```python
from build123d import *

# Parameters (mm, degrees)
SKETCH_1_R      = 2.1
EXTRUDE_1_DEPTH = 10


with BuildPart() as part:
    # 스케치1 → 보스-돌출1 (new body)
    with BuildSketch(Plane(origin=(0, 0, 0), x_dir=(1, 0, 0), z_dir=(0, 1, 0))):
        with BuildLine():
            Line((2, -4), (-2, -4))
            Line((-2, -4), (-5, -7))
            Line((-5, -7), (-5, -7.5))
            ThreePointArc((-5, -7.5), (-4.853553391, -7.853553391), (-4.5, -8))
            Line((-4.5, -8), (-3.1, -8))
            ThreePointArc((-3.1, -8), (-2.746446609, -8.146446609), (-2.6, -8.5))
            Line((-2.6, -8.5), (-2.6, -9.5))
            Line((-2.6, -9.5), (-3.1, -9.5))
            Line((-3.1, -9.5), (-3.1, -10))
            Line((-3.1, -10), (-9, -10))
            ThreePointArc((-9, -10), (-9.382683432, -9.923879533), (-9.707106781, -9.707106781))
            ThreePointArc((-9.707106781, -9.707106781), (-9.923879533, -9.382683432), (-10, -9))
            Line((-10, -9), (-10, -3.1))
            Line((-10, -3.1), (-9.5, -3.1))
            Line((-9.5, -3.1), (-9.5, -2.6))
            Line((-9.5, -2.6), (-8.5, -2.6))
            ThreePointArc((-8.5, -2.6), (-8.146446609, -2.746446609), (-8, -3.1))
            Line((-8, -3.1), (-8, -4.5))
            ThreePointArc((-8, -4.5), (-7.853553391, -4.853553391), (-7.5, -5))
            Line((-7.5, -5), (-7, -5))
            Line((-7, -5), (-4, -2))
            Line((-4, -2), (-4, 2))
            Line((-4, 2), (-7, 5))
            Line((-7, 5), (-7.5, 5))
            ThreePointArc((-7.5, 5), (-7.853553391, 4.853553391), (-8, 4.5))
            Line((-8, 4.5), (-8, 3.1))
            ThreePointArc((-8, 3.1), (-8.146446609, 2.746446609), (-8.5, 2.6))
            Line((-8.5, 2.6), (-9.5, 2.6))
            Line((-9.5, 2.6), (-9.5, 3.1))
            Line((-9.5, 3.1), (-10, 3.1))
            Line((-10, 3.1), (-10, 9))
            ThreePointArc((-10, 9), (-9.923879533, 9.382683432), (-9.707106781, 9.707106781))
            ThreePointArc((-9.707106781, 9.707106781), (-9.382683432, 9.923879533), (-9, 10))
            Line((-9, 10), (-3.1, 10))
            Line((-3.1, 10), (-3.1, 9.5))
            Line((-3.1, 9.5), (-2.6, 9.5))
            Line((-2.6, 9.5), (-2.6, 8.5))
            ThreePointArc((-2.6, 8.5), (-2.746446609, 8.146446609), (-3.1, 8))
            Line((-3.1, 8), (-4.5, 8))
            ThreePointArc((-4.5, 8), (-4.853553391, 7.853553391), (-5, 7.5))
            Line((-5, 7.5), (-5, 7))
            Line((-5, 7), (-2, 4))
            Line((-2, 4), (2, 4))
            Line((2, 4), (5, 7))
            Line((5, 7), (5, 7.5))
            ThreePointArc((5, 7.5), (4.853553391, 7.853553391), (4.5, 8))
            Line((4.5, 8), (3.1, 8))
            ThreePointArc((3.1, 8), (2.746446609, 8.146446609), (2.6, 8.5))
            Line((2.6, 8.5), (2.6, 9.5))
            Line((2.6, 9.5), (3.1, 9.5))
            Line((3.1, 9.5), (3.1, 10))
            Line((3.1, 10), (9, 10))
            ThreePointArc((9, 10), (9.382683432, 9.923879533), (9.707106781, 9.707106781))
            ThreePointArc((9.707106781, 9.707106781), (9.923879533, 9.382683432), (10, 9))
            Line((10, 9), (10, 3.1))
            Line((10, 3.1), (9.5, 3.1))
            Line((9.5, 3.1), (9.5, 2.6))
            Line((9.5, 2.6), (8.5, 2.6))
            ThreePointArc((8.5, 2.6), (8.146446609, 2.746446609), (8, 3.1))
            Line((8, 3.1), (8, 4.5))
            ThreePointArc((8, 4.5), (7.853553391, 4.853553391), (7.5, 5))
            Line((7.5, 5), (7, 5))
            Line((7, 5), (4, 2))
            Line((4, 2), (4, -2))
            Line((4, -2), (7, -5))
            Line((7, -5), (7.5, -5))
            ThreePointArc((7.5, -5), (7.853553391, -4.853553391), (8, -4.5))
            Line((8, -4.5), (8, -3.1))
            ThreePointArc((8, -3.1), (8.146446609, -2.746446609), (8.5, -2.6))
            Line((8.5, -2.6), (9.5, -2.6))
            Line((9.5, -2.6), (9.5, -3.1))
            Line((9.5, -3.1), (10, -3.1))
            Line((10, -3.1), (10, -9))
            ThreePointArc((10, -9), (9.923879533, -9.382683432), (9.707106781, -9.707106781))
            ThreePointArc((9.707106781, -9.707106781), (9.382683432, -9.923879533), (9, -10))
            Line((9, -10), (3.1, -10))
            Line((3.1, -10), (3.1, -9.5))
            Line((3.1, -9.5), (2.6, -9.5))
            Line((2.6, -9.5), (2.6, -8.5))
            ThreePointArc((2.6, -8.5), (2.746446609, -8.146446609), (3.1, -8))
            Line((3.1, -8), (4.5, -8))
            ThreePointArc((4.5, -8), (4.853553391, -7.853553391), (5, -7.5))
            Line((5, -7.5), (5, -7))
            Line((5, -7), (2, -4))
        make_face()
        Circle(SKETCH_1_R, mode=Mode.SUBTRACT)
    extrude(amount=EXTRUDE_1_DEPTH)


solid = part.part
```
Model file for the job. Use its own axes, mm. A direction names the side the tool comes from. Coordinates: 2 decimals unless noted, no trailing zeros. Loops run counter-clockwise (first coordinate to the right, second up) from the corner with the lowest first, then second, coordinate; pieces in that order, holes last. Notation, with made-up numbers: (44.25, 70) -> (85.25, 70) arc R22 ccw to (85.25, 93) -> close; hole circle Ø8 at (42.25, -28). An arc over 180 degrees is marked (long way). Answer as a JSON object with one key per item and string values.
Q1. Cut at B-B (x = 1.25). List the corners of the cut face in (y, z).
Report:
{"outline": "(0, -4) -> (10, -4) -> (10, -1.69) -> (0, -1.69) -> close; (0, 1.69) -> (10, 1.69) -> (10, 4) -> (0, 4) -> close"}
Q2. Probe probe 1 along X at (y, z) = (5.25, 0); probe 2 along X at (y, z) = (2, -3.25). List the from-to ranges inside material, lowest first.
Report:
{"probe 1": "x = -4 to -2.1, 2.1 to 4", "probe 2": "x = -10 to -8, -5.25 to 5.25, 8 to 10"}
Q3. Cut at A-A (z = 5.5). List the corners of the cut face in (x, y), and give its area (3 significant figures).
Report:
{"outline": "(-10, 0) -> (-3.5, 0) -> (-3.5, 10) -> (-10, 10) -> close; (3.5, 0) -> (10, 0) -> (10, 10) -> (3.5, 10) -> close", "area": "130 mm2"}
Q4. 3-axis set-ups, long thin cutter, end or side, ignore diameter. For faces 4 (the flat face through (9, 5, 2.6)), 5 (the flat face through (-4, 5, 8)), 6 (the flat face through (0, 5, -4)): which of +Z, -Z, +X, -X, +Y, -Y reach the whole face in a straight line?
Report:
{"face 4": "+X, +Y, -Y", "face 5": "+Y, -Y", "face 6": "-Z, +Y, -Y"}
Q5. Flat gauge pins, fed straight in: P1, Ø1.5, axis at x = -1.5, y = 3.5, coming from the -Z side; P2, Ø3, axis at y = 6.5, z = 1, coming from the -X side. Where does each tip first touch, or does it go through?
Report:
{"P1": "stops at z = -4.25", "P2": "stops at x = -4.5"}
Q6. Pull direction Z, two halves, no side cores. Call faces 1 (the flat face through (-2.6, 5, -9)), 2 (the flat face through (8, 5, -4)), 3 (the flat face through (6, 5, -10)): released by +Z, released by -Z, zero draft, split by the parting line, or undercut.
Report:
{"face 1": "zero draft", "face 2": "undercut", "face 3": "released by -Z"}
